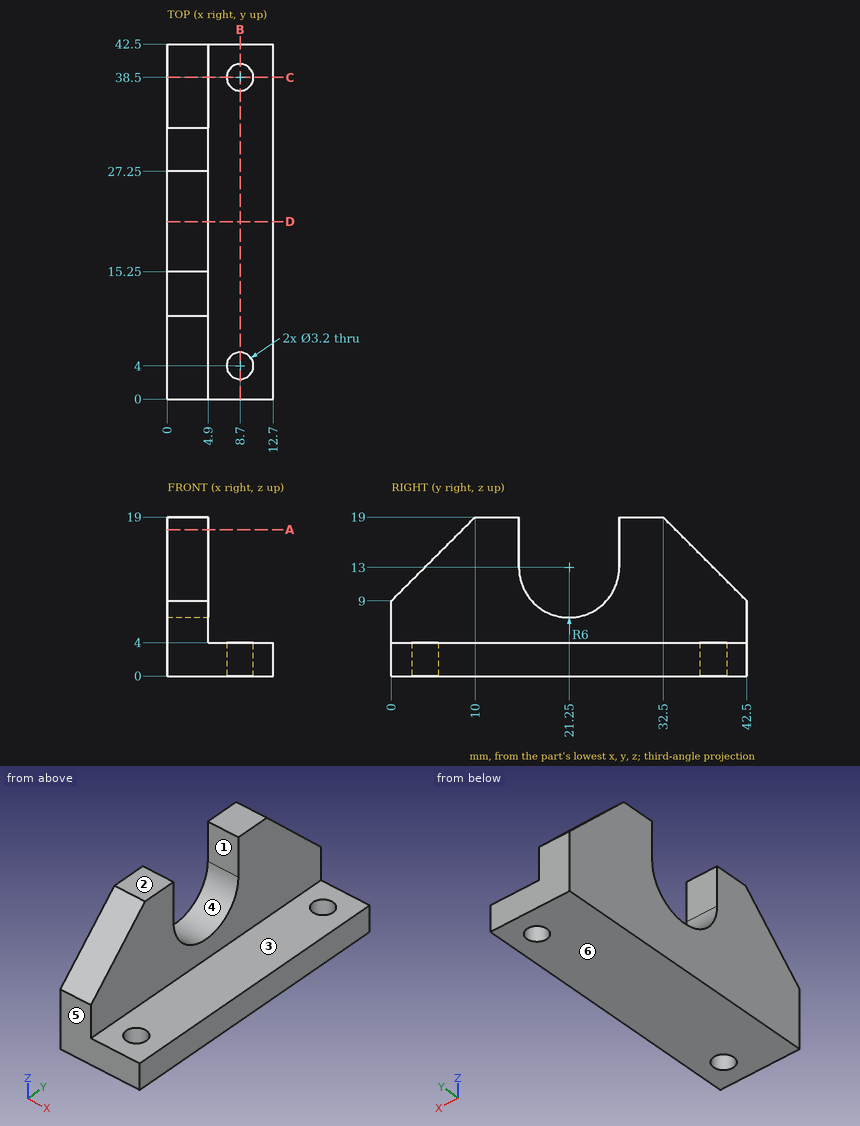
Check sheet for the drawn part. Datum: minimum x, y, z corner. Units: mm. A direction names the side the tool comes from. Round coordinates to 2 decimals unless told otherwise and drop trailing zeros. Write each loop counter-clockwise with the first axis right and the second up, starting at its lowest first coordinate (ties: lowest second). Pieces come first, ordered by that corner, then holes. Notation, with made-up numbers: (31, 55) - (85, 55) arc R21 ccw to (85, 68) - close; hole circle Ø1 at (-7.75, 59). An arc over 180 degrees is marked (long way). Return JSON: item names as keys, results as strings.
Q1. Scan lines: L1, parallel to Y at x = 8.7, z = 2.4; L2, parallel to Y at x = 9.75, z = 2.75; L3, parallel to Z at x = 9.75, y = 10. Record each from-to range of solid material in increasing order. Write a range as from..to.
Returned:
{"L1": "y = 0..2.4, 5.6..36.9, 40.1..42.5", "L2": "y = 0..2.79, 5.21..37.29, 39.71..42.5", "L3": "z = 0..4"}
Q2. Draft check along Y on the marked faces 4, 5 and 6. Enter one of: released by +Y, released by -Y, zero draft, split by the parting line, or undercut.
Returned:
{"face 4": "undercut", "face 5": "released by -Y", "face 6": "zero draft"}
Q3. Cross-section at B-B (x = 8.7). Record the boundary of the cut face in (y, z), then the cut area to 3 significant figures.
Returned:
{"outline": "(0, 0) - (2.4, 0) - (2.4, 4) - (0, 4) - close; (5.6, 0) - (36.9, 0) - (36.9, 4) - (5.6, 4) - close; (40.1, 0) - (42.5, 0) - (42.5, 4) - (40.1, 4) - close", "area": "144 mm²"}
Q4. Cross-section at C-C (y = 38.5). Record the boundary of the cut face in (x, z).
Returned:
{"outline": "(0, 0) - (7.1, 0) - (7.1, 4) - (4.9, 4) - (4.9, 13) - (0, 13) - close; (10.3, 0) - (12.7, 0) - (12.7, 4) - (10.3, 4) - close"}
Q5. Depth check by flat-ended pin: P1, Ø6, axis at x = 7, z = 7.5, coming from the +Y side; P2, Ø7.5, axis at y = 22.5, z = 12, coming from the +X side; P3, Ø2, axis at x = 7, y = 33, coming from the +Z side; P4, Ø4, axis at x = 3, z = 16.5, coming from the -Y side. Enter the tip coordinate at first touch or a pass-through.
Returned:
{"P1": "stops at y = 42.5", "P2": "passes through", "P3": "stops at z = 4", "P4": "stops at y = 5.5"}
Q6. Cross-section at A-A (z = 17.5). Record the boundary of the cut face in (x, y).
Returned:
{"outline": "(0, 8.5) - (4.9, 8.5) - (4.9, 15.25) - (0, 15.25) - close; (0, 27.25) - (4.9, 27.25) - (4.9, 34) - (0, 34) - close"}
Q7. Access from +Z, -Z, +X, -X, +Y, -Y to the whole of each face (thin tool, end or side, straight path). Record for the marked faces 1, 2 and 3.
Returned:
{"face 1": "+Z, +X, -X", "face 2": "+Z, +X, -X, +Y, -Y", "face 3": "+Z, +X, +Y, -Y"}
Q8. Cross-section at D-D (y = 21.25). Record the boundary of the cut face in (x, z).
Returned:
{"outline": "(0, 0) - (12.7, 0) - (12.7, 4) - (4.9, 4) - (4.9, 7) - (0, 7) - close"}
